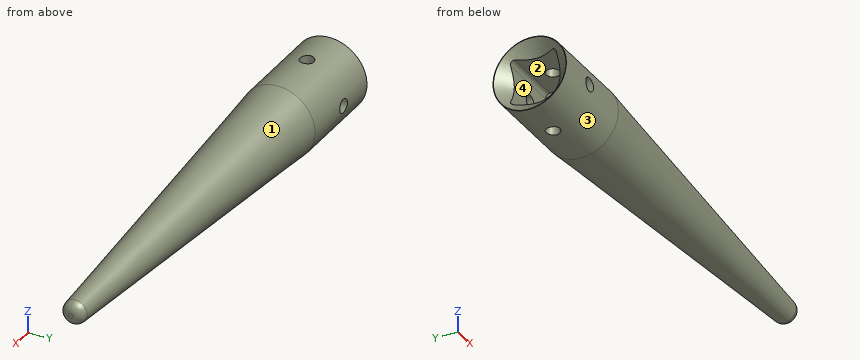
from build123d import *

# Parameters (mm, degrees)
ENL_V_MAT_EXTRU_1_DEPTH      = 15
ESQUISSE3_R                  = 1.5
ENL_V_MAT_EXTRU_2_DEPTH      = 9
ENL_V_MAT_EXTRU_2_DEPTH_BACK = 9
ESQUISSE4_R                  = 1.5
ENL_V_MAT_EXTRU_3_DEPTH      = 9.0000001
ENL_V_MAT_EXTRU_3_DEPTH_BACK = 9.0000001


with BuildPart() as part:
    # Esquisse1 → Révolution1 (revolve)
    with BuildSketch(Plane.XY, mode=Mode.PRIVATE) as r_volution1_sk:
        with BuildLine():
            Line((7.9, 0), (0, 7.9))
            Line((0, 7.9), (0, 8))
            Line((0, 8), (20, 8))
            Line((20, 8), (98.139512947, 2.535952973))
            ThreePointArc((98.139512947, 2.535952973), (99.462707403, 1.904821592), (100, 0.540824872))
            Line((100, 0.540824872), (100, 0))
            Line((100, 0), (7.9, 0))
        make_face()
    revolve(r_volution1_sk.sketch.rotate(Axis((0, 0, 0), (1, 0, 0)), 90), axis=Axis((0, 0, 0), (1, 0, 0)))  # turned: the seam where the file's is

    # Esquisse2 → Enlèv. mat.-Extru.1 (cut)
    with BuildSketch(Plane(origin=(0, 0, 0), x_dir=(0, 0, -1), z_dir=(1, 0, 0))):
        with BuildLine():
            Line((4, 5), (-4, 5))
            ThreePointArc((-4, 5), (-4.707106781, 4.707106781), (-5, 4))
            Line((-5, 4), (-5, -4))
            ThreePointArc((-5, -4), (-4.707106781, -4.707106781), (-4, -5))
            Line((-4, -5), (4, -5))
            ThreePointArc((4, -5), (4.707106781, -4.707106781), (5, -4))
            Line((5, -4), (5, 4))
            ThreePointArc((5, 4), (4.707106781, 4.707106781), (4, 5))
        make_face()
    extrude(amount=ENL_V_MAT_EXTRU_1_DEPTH, mode=Mode.SUBTRACT)

    # Esquisse3 → Enlèv. mat.-Extru.2 (cut, two sides)
    with BuildSketch(Plane(origin=(0, 0, 0), x_dir=(1, 0, 0), z_dir=(0, 1, 0))) as enl_v_mat_extru_2_sk:
        with Locations(Location((9, 0, 0), (0, 0, 270))):  # turned: the seam where the file's is
            Circle(ESQUISSE3_R)
    extrude(amount=ENL_V_MAT_EXTRU_2_DEPTH, mode=Mode.SUBTRACT)
    extrude(enl_v_mat_extru_2_sk.sketch, amount=-ENL_V_MAT_EXTRU_2_DEPTH_BACK, mode=Mode.SUBTRACT)

    # Esquisse4 → Enlèv. mat.-Extru.3 (cut, two sides)
    with BuildSketch(Plane.XY) as enl_v_mat_extru_3_sk:
        with Locations((9, 0)):
            Circle(ESQUISSE4_R)
    extrude(amount=ENL_V_MAT_EXTRU_3_DEPTH, mode=Mode.SUBTRACT)
    extrude(enl_v_mat_extru_3_sk.sketch, amount=-ENL_V_MAT_EXTRU_3_DEPTH_BACK, mode=Mode.SUBTRACT)


solid = part.part
Verification items for the finished model (mm, model axes). Face numbers are marked on the shaded views. A direction names the side the tool comes from. Round coordinates to 2 decimals unless told otherwise and drop trailing zeros. Loops run counter-clockwise (first coordinate to the right, second up) from the corner with the lowest first, then second, coordinate; pieces in that order, holes last. Notation, with made-up numbers: M 42,49 L 98,49 A12 cw 98,58 Z; hole C -26.5,55 d6. An arc over 180 degrees is marked long. Write each question's results on one line, items separated by ' | '.
1) Access from +Z, -Z, +X, -X, +Y, -Y to the whole of each face (thin tool, end or side, straight path). Record for the marked faces 3 and 4.
Checks:
face 3: +X, -X | face 4: -X
2) Scan lines: L1, parallel to Z at x = 9, y = -5.6; L2, parallel to Z at x = 9, y = -6.95; L3, parallel to Y at x = 9, z = -7.35. Record each from-to range of solid material in increasing order. Write a range as from..to.
Checks:
L1: z = -5.71..-1.5, 1.5..5.71 | L2: z = -3.96..-1.5, 1.5..3.96 | L3: y = -3.16..-1.5, 1.5..3.16
3) Section check B-B on x = 92. Record the boundary of the cut face in (y, z).
Checks:
outline: C 0,0 d5.93
4) Mould release check, pull along Z, two halves, no side actions. Record for the marked faces 1 and 2: released by +Z, released by -Z, zero draft, split by the parting line, or undercut.
Checks:
face 1: split by the parting line | face 2: undercut
5) Gauge pin test, flat ends, axial feed: P1, Ø1.8, axis at x = 9, z = 0, coming from the +Y side; P2, Ø1, axis at x = 18, y = 0.5, coming from the +Z side; P3, Ø1, axis at x = 73, z = 0, coming from the -Y side; P4, Ø8, axis at y = -0.5, z = -0.5, coming from the -X side. Record the tip position at first contact, or that the pin passes through.
Checks:
P1: passes through | P2: stops at z = 8 | P3: stops at y = -4.33 | P4: stops at x = 15
6) Section check A-A on x = 9. Record the boundary of the cut face in (y, z), then the cut area to 3 significant figures.
Checks:
outline: M -7.86,-1.5 A8 ccw -1.5,-7.86 L -1.5,-5 L -4,-5 A1 cw -5,-4 L -5,-1.5 Z; M -7.86,1.5 L -5,1.5 L -5,4 A1 cw -4,5 L -1.5,5 L -1.5,7.86 A8 ccw Z; M 1.5,-7.86 A8 ccw 7.86,-1.5 L 5,-1.5 L 5,-4 A1 cw 4,-5 L 1.5,-5 Z; M 1.5,5 L 4,5 A1 cw 5,4 L 5,1.5 L 7.86,1.5 A8 ccw 1.5,7.86 Z | area: 66.5 mm2
